Check sheet for the modelled part. Datum: model origin and axes. Units: mm. A direction names the side the tool comes from. Round coordinates to 2 decimals unless told otherwise and drop trailing zeros. Loops run counter-clockwise (first coordinate to the right, second up) from the corner with the lowest first, then second, coordinate; pieces in that order, holes last. Notation, with made-up numbers: (85.5, 23.5) - (122.5, 23.5) arc R14 cw to (122.5, 37.5) - close; hole circle Ø9 at (76.25, 9). An arc over 180 degrees is marked (long way). Put each result on its own line as item: value. Start each with the question number.
Item 1: Section check C-C, the plane y = -31.75. Record the cut outline in (x, z), and give its area (3 significant figures).
Item 2: Section check B-B, the plane x = -10. Record the cut outline in (y, z).
Item 3: Tool access check on faces 4 (the flat face through (9, -38, -3.528)), 5 (the flat face through (6.35, -38, 11)), 6 (the flat face through (7, -50.8, 5)). Record the directions out of +Z, -Z, +X, -X, +Y, -Y that give a thin tool (end or side, any length) a straight path to the whole face; none if there is none.
Item 4: Draft check along X on faces 1 (the flat face through (-16.642, -38, 0)), 2 (the flat face through (7, -25.4, 5)), 3 (the flat face through (6.35, -38, -11)). Enter one of: pulls with the +X half, pulls with the -X half, needs draft (parallel to the pull), parting line crosses it, or undercut.
Item 5: Section check D-D, the plane z = 1.5. Record the cut outline in (x, y), and give its area (3 significant figures).
Item 6: Section check A-A, the plane z = -13. Record the cut outline in (x, y), and give its area (3 significant figures).
Item 7: Material ranges on line 1 along Z through (x, y) = (7, -38.5); line 2 along Z through (x, y) = (-2.5, -32); line 3 along X through (y, z) = (-40.25, 13), recorded low to high.
from build123d import *

# Parameters (mm, degrees)
F2_DEPTH = 25.4


with BuildPart() as f2:
    # F1 (on offset) → F2 (new body)
    with BuildSketch(Plane.XZ.offset(25.4)):
        Polygon((-12.7, -19.402778), (-12.7, 18.697222), (6.35, 18.697222), (6.35, 2.822222), (11.678541, 2.822222), (11.678541, 22.919137), (-16.641926, 22.919137), (-16.641926, -24.378963), (11.678541, -24.378963), (11.678541, -3.527778), (6.35, -3.527778), (6.35, -19.402778), align=None)
    extrude(amount=F2_DEPTH)


solid = f2.part
Check result:
1. outline: (-16.64, -24.38) - (11.68, -24.38) - (11.68, -3.53) - (6.35, -3.53) - (6.35, -19.4) - (-12.7, -19.4) - (-12.7, 18.7) - (6.35, 18.7) - (6.35, 2.82) - (11.68, 2.82) - (11.68, 22.92) - (-16.64, 22.92) - close
1. area: 580 mm²
2. outline: (-50.8, -24.38) - (-25.4, -24.38) - (-25.4, -19.4) - (-50.8, -19.4) - close; (-50.8, 18.7) - (-25.4, 18.7) - (-25.4, 22.92) - (-50.8, 22.92) - close
3. face 4: +X, +Y, -Y
3. face 5: +Y, -Y
3. face 6: +Z, -Z, +X, -X, -Y
4. face 1: pulls with the -X half
4. face 2: needs draft
4. face 3: undercut
5. outline: (-16.64, -50.8) - (-12.7, -50.8) - (-12.7, -25.4) - (-16.64, -25.4) - close
5. area: 100 mm²
6. outline: (-16.64, -50.8) - (-12.7, -50.8) - (-12.7, -25.4) - (-16.64, -25.4) - close; (6.35, -50.8) - (11.68, -50.8) - (11.68, -25.4) - (6.35, -25.4) - close
6. area: 235 mm²
7. line 1: -24.38 to -3.53, 2.82 to 22.92
7. line 2: -24.38 to -19.4, 18.7 to 22.92
7. line 3: -16.64 to -12.7, 6.35 to 11.68
